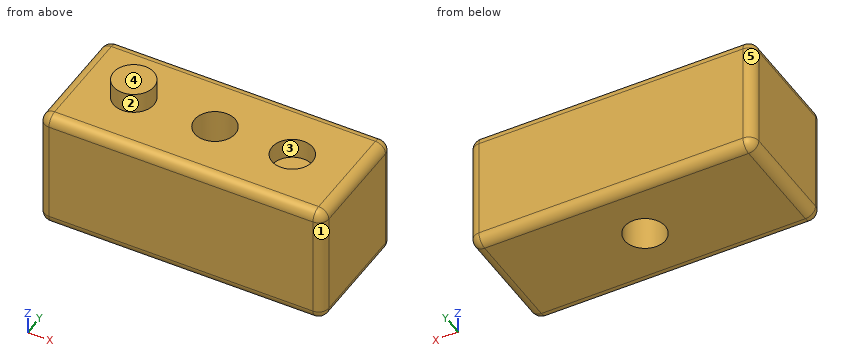
```python
from build123d import *

# Parameters (mm, degrees)
F0_W     = 140
F0_H     = 60
F1_DEPTH = 60
F2_R     = 10
F5_DEPTH = 10
F3_R     = 10
F6_DEPTH = 10
F4_R     = 10
F7_DEPTH = 877
F8_R     = 5


with BuildPart() as f1:
    # F0 (on Top) → F1 (new body)
    with BuildSketch(Plane.XY):
        Rectangle(F0_W, F0_H)
    extrude(amount=F1_DEPTH)

    # F2 (on face) → F5 (join)
    with BuildSketch(Plane.XY.offset(60)):
        with Locations((-40, 0)):
            Circle(F2_R)
    extrude(amount=F5_DEPTH)

    # F3 (on face) → F6 (cut)
    with BuildSketch(Plane.XY.offset(60)):
        with Locations((38.061067, 0)):
            Circle(F3_R)
    extrude(amount=-F6_DEPTH, mode=Mode.SUBTRACT)

    # F4 (on face) → F7 (cut)
    with BuildSketch(Plane.XY.offset(60)):
        Circle(F4_R)
    extrude(amount=-F7_DEPTH, mode=Mode.SUBTRACT)

    # F8
    f8_edges = [f1.edges().sort_by_distance(p)[0] for p in [
        (0, -30, 60),
        (0, 30, 60),
        (-70, 0, 60),
        (70, 0, 60),
        (-70, -30, 30),
        (-70, 30, 30),
        (-70, 0, 0),
        (70, -30, 30),
        (70, 0, 0),
        (70, 30, 30),
        (0, -30, 0),
        (0, 30, 0),
    ]]
    fillet(f8_edges, radius=F8_R)


solid = f1.part
```
Design review of the part built by this model. Coordinates are the model's own, in mm. Face numbers are marked on the shaded views. A direction names the side the tool comes from. Coordinates: 2 decimals unless noted, no trailing zeros. Write each loop counter-clockwise with the first axis right and the second up, starting at its lowest first coordinate (ties: lowest second). Pieces come first, ordered by that corner, then holes. Notation, with made-up numbers: M 62.5,28.5 L 96.5,28.5 A25 ccw 96.5,52.5 Z; hole C 19,34 d9. An arc over 180 degrees is marked long. Answer as a JSON object with one key per item and string values.
Item 1: Machinability: for the marked faces 1 and 2, which of the approach directions +Z, -Z, +X, -X, +Y, -Y give a long, thin tool a straight path to every point of the face, cutting with its end or side? Answer none if there is none.
Outcome:
{"face 1": "+Z, -Z, +X, -Y", "face 2": "+Z"}
Item 2: Add section A-A, the plane x = 0. Give the boundary of the cut face in (y, z).
Outcome:
{"outline": "M -30,5 A5 ccw -25,0 L -10,0 L -10,60 L -25,60 A5 ccw -30,55 Z; M 10,0 L 25,0 A5 ccw 30,5 L 30,55 A5 ccw 25,60 L 10,60 Z"}
Item 3: Insertion check: pin 1 Ø1.5 at (x, y) = (-47, -13) entering from +Z; pin 2 Ø16 at (x, y) = (38.06, 0) entering from +Z; pin 3 Ø2 at (y, z) = (3, 61.5) entering from +X. Each pin has a flat end and moves straight along its axis. Give the tip position at first contact, or say it passes through.
Outcome:
{"pin 1": "z = 60", "pin 2": "z = 50", "pin 3": "x = -30.2"}
Item 4: Add section B-B, the plane y = 0. Give the boundary of the cut face in (x, z).
Outcome:
{"outline": "M -70,5 A5 ccw -65,0 L -10,0 L -10,60 L -30,60 L -30,70 L -50,70 L -50,60 L -65,60 A5 ccw -70,55 Z; M 10,0 L 65,0 A5 ccw 70,5 L 70,55 A5 ccw 65,60 L 48.06,60 L 48.06,50 L 28.06,50 L 28.06,60 L 10,60 Z"}
Item 5: Add section C-C, the plane z = 12. Give the boundary of the cut face in (x, y).
Outcome:
{"outline": "M -70,-25 A5 ccw -65,-30 L 65,-30 A5 ccw 70,-25 L 70,25 A5 ccw 65,30 L -65,30 A5 ccw -70,25 Z; hole C 0,0 d20"}
Item 6: Add section D-D, the plane y = -20. Give the boundary of the cut face in (x, z), and give its area (3 significant figures).
Outcome:
{"outline": "M -70,5 A5 ccw -65,0 L 65,0 A5 ccw 70,5 L 70,55 A5 ccw 65,60 L -65,60 A5 ccw -70,55 Z", "area": "8,380 mm²"}
Item 7: Draft analysis for pull direction X (two halves, no side actions). For the marked faces 3, 4 and 5, state which applies: pulls with the +X half, pulls with the -X half, needs draft (parallel to the pull), parting line crosses it, or undercut.
Outcome:
{"face 3": "undercut", "face 4": "needs draft", "face 5": "pulls with the -X half"}
Item 8: Wall thickness on probe 1 along Y at (x, z) = (0, 26); probe 2 along X at (y, z) = (2.5, 56); probe 3 along Z at (x, y) = (-61, 18): over which ranges is each line inside the solid? List them lowest first.
Outcome:
{"probe 1": "-30 to -10, 10 to 30", "probe 2": "-69.9 to -9.68, 9.68 to 28.38, 47.74 to 69.9", "probe 3": "0 to 60"}
